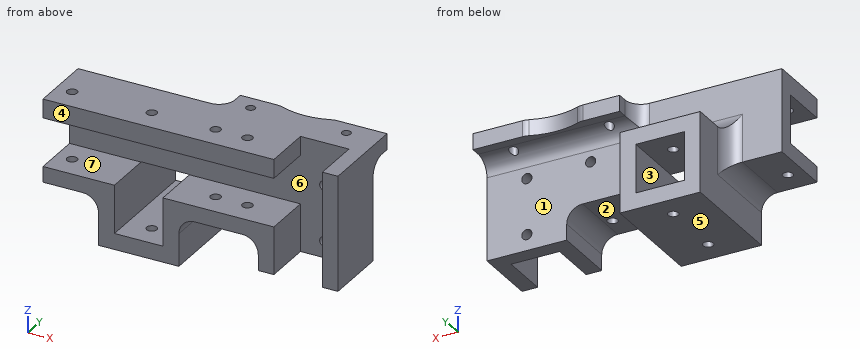
```python
from build123d import *

# Parameters (mm, degrees)
SKETCH_1_W          = 15.2
SKETCH_1_H          = 15.2
EXTRUDE_1_DEPTH     = 20
SKETCH_2_W          = 25.2
SKETCH_2_H          = 25.2
SKETCH_2_W_2        = 15.2
SKETCH_2_H_2        = 15.2
EXTRUDE_2_DEPTH     = 15
SKETCH_3_W          = 15.2
SKETCH_3_H          = 15.2
CUT_EXTRUDE_1_DEPTH = 80
SKETCH_4_R          = 1.6
CUT_EXTRUDE_2_DEPTH = 83.635888087
FILLET_1_R          = 5
SKETCH_5_W          = 15.2
SKETCH_5_H          = 15.2
CUT_EXTRUDE_3_DEPTH = 83.635888087
CUT_EXTRUDE_5_REACH = 73.229
SKETCH_7_R          = 1.6
SKETCH_8_W          = 46
SKETCH_8_H          = 5
EXTRUDE_3_DEPTH     = 8
FILLET_2_R          = 5
CUT_EXTRUDE_6_REACH = 84.636
SKETCH_9_R          = 21.25
SKETCH_9_R_2        = 1.4
FILLET_3_R          = 5


with BuildPart() as part:
    # 草图1 → 凸台-拉伸1 (new body)
    with BuildSketch(Plane(origin=(0, 0, 0), x_dir=(1, 0, 0), z_dir=(0, 1, 0))):
        Polygon((-30, 12.5), (-12.6, 12.5), (-12.6, 27.7), (12.6, 27.7), (12.6, 12.5), (37.5, 12.5), (37.5, 22.5), (62.5, 22.5), (62.5, -13.5), (-30, -13.5), align=None)
        with Locations((0, 15.1)):
            Rectangle(SKETCH_1_W, SKETCH_1_H, mode=Mode.SUBTRACT)
    extrude(amount=EXTRUDE_1_DEPTH)

    # 草图2 → 凸台-拉伸2 (add)
    with BuildSketch(Plane(origin=(0, 20, 0), x_dir=(1, 0, 0), z_dir=(0, 1, 0))):
        with Locations((0, 15.1)):
            Rectangle(SKETCH_2_W, SKETCH_2_H)
        with Locations((0, 15.1)):
            Rectangle(SKETCH_2_W_2, SKETCH_2_H_2, mode=Mode.SUBTRACT)
    extrude(amount=EXTRUDE_2_DEPTH)

    # 草图3 → 切除-拉伸1 (cut)
    with BuildSketch(Plane(origin=(-30, 0, 0), x_dir=(0, 0, -1), z_dir=(1, 0, 0))):
        with Locations((0, 7.6)):
            Rectangle(SKETCH_3_W, SKETCH_3_H)
    extrude(amount=CUT_EXTRUDE_1_DEPTH, mode=Mode.SUBTRACT)

    # 草图4 → 切除-拉伸2 (cut, through all)
    with BuildSketch(Plane.XY.offset(13.5)):
        with Locations((0, 7.5)):
            Circle(SKETCH_4_R)
        with Locations((20, 7.5)):
            Circle(SKETCH_4_R)
        with Locations((-25, 7.5)):
            Circle(SKETCH_4_R)
        with Locations((0, 27.5)):
            Circle(SKETCH_4_R)
        with Locations((30, 7.5)):
            Circle(SKETCH_4_R)
    extrude(amount=-CUT_EXTRUDE_2_DEPTH, mode=Mode.SUBTRACT)

    # 圆角1
    fillet_1_edges = [part.edges().sort_by_distance(p)[0] for p in [
        (-12.6, 10, -12.5),
        (12.6, 10, -12.5),
        (37.5, 10, -12.5),
        (-12.6, 20, -7.5),
        (0, 20, -2.5),
        (12.6, 20, -7.5),
    ]]
    fillet(fillet_1_edges, radius=FILLET_1_R)

    # 草图5 → 切除-拉伸3 (cut, through all)
    with BuildSketch(Plane.XY.offset(13.5)):
        with Locations((50, 7.6)):
            Rectangle(SKETCH_5_W, SKETCH_5_H)
    extrude(amount=-CUT_EXTRUDE_3_DEPTH, mode=Mode.SUBTRACT)

    # 草图7 → 切除-拉伸5 (cut, up to next)
    with BuildSketch(Plane(origin=(0, 20, 0), x_dir=(1, 0, 0), z_dir=(0, 1, 0)), mode=Mode.PRIVATE) as cut_extrude_5_sk1:
        with Locations(Location((50, 0, 0), (0, 0, 270))):
            Circle(SKETCH_7_R)
    cut_extrude_5_tool1 = extrude(cut_extrude_5_sk1.sketch, amount=-CUT_EXTRUDE_5_REACH, mode=Mode.PRIVATE) & part.part
    # 草图7 → 切除-拉伸5 (cut, up to next)
    with BuildSketch(Plane(origin=(0, 20, 0), x_dir=(1, 0, 0), z_dir=(0, 1, 0)), mode=Mode.PRIVATE) as cut_extrude_5_sk2:
        with Locations(Location((30, 0, 0), (0, 0, 270))):
            Circle(SKETCH_7_R)
    cut_extrude_5_tool2 = extrude(cut_extrude_5_sk2.sketch, amount=-CUT_EXTRUDE_5_REACH, mode=Mode.PRIVATE) & part.part
    # 草图7 → 切除-拉伸5 (cut, up to next)
    with BuildSketch(Plane(origin=(0, 20, 0), x_dir=(1, 0, 0), z_dir=(0, 1, 0)), mode=Mode.PRIVATE) as cut_extrude_5_sk3:
        with Locations(Location((50, 17.5, 0), (0, 0, 270))):
            Circle(SKETCH_7_R)
    cut_extrude_5_tool3 = extrude(cut_extrude_5_sk3.sketch, amount=-CUT_EXTRUDE_5_REACH, mode=Mode.PRIVATE) & part.part
    add(cut_extrude_5_tool1.solids().sort_by_distance((50, 20, 0))[0], mode=Mode.SUBTRACT)
    add(cut_extrude_5_tool2.solids().sort_by_distance((30, 20, 0))[0], mode=Mode.SUBTRACT)
    add(cut_extrude_5_tool3.solids().sort_by_distance((50, 20, -17.5))[0], mode=Mode.SUBTRACT)

    # 草图8 → 凸台-拉伸3 (add)
    with BuildSketch(Plane(origin=(0, 20, 0), x_dir=(1, 0, 0), z_dir=(0, 1, 0))):
        with Locations((39.5, -11)):
            Rectangle(SKETCH_8_W, SKETCH_8_H)
    extrude(amount=EXTRUDE_3_DEPTH)

    # 圆角2
    fillet_2_edges = [part.edges().sort_by_distance(p)[0] for p in [
        (39.5, 20, 8.5),
    ]]
    fillet(fillet_2_edges, radius=FILLET_2_R)

    # 草图9 → 切除-拉伸6 (cut, up to next)
    with BuildSketch(Plane.XY.offset(13.5), mode=Mode.PRIVATE) as cut_extrude_6_sk1:
        with Locations((37.5, 47.5)):
            Circle(SKETCH_9_R)
    cut_extrude_6_tool1 = extrude(cut_extrude_6_sk1.sketch, amount=-CUT_EXTRUDE_6_REACH, mode=Mode.PRIVATE) & part.part
    # 草图9 → 切除-拉伸6 (cut, up to next)
    with BuildSketch(Plane.XY.offset(13.5), mode=Mode.PRIVATE) as cut_extrude_6_sk2:
        with Locations((22.5, 23)):
            Circle(SKETCH_9_R_2)
    cut_extrude_6_tool2 = extrude(cut_extrude_6_sk2.sketch, amount=-CUT_EXTRUDE_6_REACH, mode=Mode.PRIVATE) & part.part
    # 草图9 → 切除-拉伸6 (cut, up to next)
    with BuildSketch(Plane.XY.offset(13.5), mode=Mode.PRIVATE) as cut_extrude_6_sk3:
        with Locations((52.5, 23)):
            Circle(SKETCH_9_R_2)
    cut_extrude_6_tool3 = extrude(cut_extrude_6_sk3.sketch, amount=-CUT_EXTRUDE_6_REACH, mode=Mode.PRIVATE) & part.part
    add(cut_extrude_6_tool1.solids().sort_by_distance((37.5, 47.5, 13.5))[0], mode=Mode.SUBTRACT)
    add(cut_extrude_6_tool2.solids().sort_by_distance((22.5, 23, 13.5))[0], mode=Mode.SUBTRACT)
    add(cut_extrude_6_tool3.solids().sort_by_distance((52.5, 23, 13.5))[0], mode=Mode.SUBTRACT)

    # 圆角3
    fillet_3_edges = [part.edges().sort_by_distance(p)[0] for p in [
        (16.5, 20, 8.5),
        (45.944672877, 28, 11),
        (29.055327123, 28, 11),
    ]]
    fillet(fillet_3_edges, radius=FILLET_3_R)


solid = part.part
```
Geometry: final body of the model. Coordinates: model frame, mm. Face numbers are marked on the shaded views. A direction names the side the tool comes from. Round coordinates to 2 decimals unless told otherwise and drop trailing zeros. Order: outer loops, then holes, each group sorted by start corner. A loop starts at its lowest first (then second) coordinate and runs counter-clockwise, first axis right, second up. Notation, with made-up numbers: (-6, 3) - (-2, 3) arc R14 ccw to (-2, 8) - close; hole circle Ø2 at (54, 50.5). An arc over 180 degrees is marked (long way). Use CSV: the item, a comma, the result in double quotes. Start each with the question number.
Q1. Section query A-A (x = -25). Return loops of the section in (y, z).
Q2. Mould query, pull axis Z, two halves, no side actions, for the marked faces 4, 5, 6 and 7. Classes: +Z half, -Z half, draft (parallel to the pull), parting line (faces both ways), or undercut.
Q3. Section query B-B (z = -21). Return loops of the section in (x, y).
Q4. Section query D-D (z = -9). Return loops of the section in (x, y), and give its area (3 significant figures).
Q5. Section query C-C (y = 3). Return loops of the section in (x, z).
Q6. First-contact query: pin 1 (5 mm diameter, centred on x = 0, y = 27.5, fed in from -Z); pin 2 (8 mm diameter, centred on y = 26.5, z = -12.5, fed in from -X); pin 3 (4 mm diameter, centred on y = 6, z = -20, fed in from -X); pin 4 (5 mm diameter, centred on x = 2, y = 30.5, fed in from +Z). Flat tips, straight axial feed; report the tip coordinate or a pass-through.
Q7. Access query for the marked faces 1, 2 and 3. Directions: +Z, -Z, +X, -X, +Y, -Y. A direction counts if a zero-diameter tool reaches every point of the face in a straight line with its end or side. Return the directions, or none.
Q8. Material intervals for line 1 along X through (y, z) = (10, -8); line 2 along Z through (x, y) = (-2.5, 19.5); line 3 along Z through (x, y) = (24, 4.5), sorted ascending. Write a range as from..to.
Result set:
1,outline,"(0, -12.5) - (5.9, -12.5) - (5.9, -7.6) - (0, -7.6) - close; (0, 7.6) - (5.9, 7.6) - (5.9, 13.5) - (0, 13.5) - close; (9.1, -12.5) - (20, -12.5) - (20, 13.5) - (9.1, 13.5) - (9.1, 7.6) - (15.2, 7.6) - (15.2, -7.6) - (9.1, -7.6) - close"
2,face 4,"draft"
2,face 5,"-Z half"
2,face 6,"undercut"
2,face 7,"undercut"
3,outline,"(-12.6, 0) - (-7.6, 0) - (-7.6, 35) - (-12.6, 35) - close; (7.6, 0) - (12.6, 0) - (12.6, 35) - (7.6, 35) - close; (37.5, 0) - (42.4, 0) - (42.4, 15.2) - (57.6, 15.2) - (57.6, 0) - (62.5, 0) - (62.5, 20) - (37.5, 20) - close"
4,outline,"(-30, 0) - (-7.6, 0) - (-7.6, 35) - (-12.6, 35) - (-12.6, 25) arc R5 cw to (-17.6, 20) - (-30, 20) - close; (7.6, 0) - (42.4, 0) - (42.4, 15.2) - (57.6, 15.2) - (57.6, 0) - (62.5, 0) - (62.5, 20) - (17.6, 20) arc R5 cw to (12.6, 25) - (12.6, 35) - (7.6, 35) - close; hole circle Ø3.2 at (-25, 7.5); hole circle Ø3.2 at (20, 7.5); hole circle Ø3.2 at (30, 7.5)"
4,area,"1,450 mm2"
5,outline,"(-30, -12.5) - (-17.6, -12.5) arc R5 cw to (-12.6, -17.5) - (-12.6, -27.7) - (12.6, -27.7) - (12.6, -17.5) arc R5 cw to (17.6, -12.5) - (32.5, -12.5) arc R5 cw to (37.5, -17.5) - (37.5, -22.5) - (42.4, -22.5) - (42.4, -7.6) - (7.6, -7.6) - (7.6, -22.7) - (-7.6, -22.7) - (-7.6, -7.6) - (-30, -7.6) - close; (-30, 7.6) - (42.4, 7.6) - (42.4, 13.5) - (-30, 13.5) - close; (57.6, -22.5) - (62.5, -22.5) - (62.5, 13.5) - (57.6, 13.5) - close"
6,pin 1,"stops at z = -27.7"
6,pin 2,"stops at x = -13.27"
6,pin 3,"stops at x = -12.6"
6,pin 4,"stops at z = -2.5"
7,face 1,"+Y"
7,face 2,"-Z, +Y, -Y"
7,face 3,"+Y, -Y"
8,line 1,"x = -30..-7.6, 7.6..42.4, 57.6..62.5"
8,line 2,"z = -27.7..-22.7, -7.5..13.5"
8,line 3,"z = -12.5..-7.6, 7.6..13.5"
